from build123d import *

# Parameters (mm, degrees)
SKETCH1_R           = 3.175
BOSS_EXTRUDE1_DEPTH = 5.5499
FILLET1_START       = -5.5499
FILLET1_DEPTH       = 11.0998
SKETCH2_R           = 2.286
SKETCH2_R_2         = 1.89865
CUT_EXTRUDE1_DEPTH  = 5.08


with BuildPart() as part:
    # Sketch1 → Boss-Extrude1 (new, symmetric)
    with BuildSketch(Plane(origin=(0, 0, 0), x_dir=(1, 0, 0), z_dir=(0, 1, 0))):
        with BuildLine():
            Line((0, 6.35), (12.366459894, 6.35))
            Line((12.366459894, 6.35), (57.15, 6.35))
            Line((57.15, 6.35), (57.15, -3.81))
            Line((57.15, -3.81), (6.35, -3.81))
            Line((6.35, -3.81), (6.35, 0))
            ThreePointArc((6.35, 0), (-4.490128061, -4.490128061), (0, 6.35))
        make_face()
        with Locations(Location((0, 0, 0), (0, 0, 270))):
            Circle(SKETCH1_R, mode=Mode.SUBTRACT)
    extrude(amount=BOSS_EXTRUDE1_DEPTH, both=True)

    # Fillet1: read off the stored shape, not the designer's step
    # Fillet1 outline → Fillet1 (add)
    with BuildSketch(Plane(origin=(0, 0, 0), x_dir=(1, 0, 0), z_dir=(0, 1, 0)).offset(FILLET1_START)):
        with BuildLine():
            ThreePointArc((4.446322142, -4.533510716), (5.322474594, -3.972611562), (6.35, -3.81))
            Line((6.35, -3.81), (6.35, 0))
            ThreePointArc((6.35, 0), (5.854769236, -2.458490838), (4.446322142, -4.533510716))
        make_face()
    extrude(amount=FILLET1_DEPTH)

    # Sketch2 → Cut-Extrude1 (cut)
    with BuildSketch(Plane.XY.offset(3.81)):
        with Locations((13.97, 1.7399)):
            Circle(SKETCH2_R)
        with Locations((49.53, 1.7399)):
            Circle(SKETCH2_R)
        with Locations((13.97, 1.7399)):
            Circle(SKETCH2_R_2)
        with Locations((49.53, 1.7399)):
            Circle(SKETCH2_R_2)
    extrude(amount=-CUT_EXTRUDE1_DEPTH, mode=Mode.SUBTRACT)


solid = part.part
Can you work these out from the model? Positions are in its coordinate system, mm. A direction names the side the tool comes from. Give positions to 0.01 mm unless a question says otherwise; leave off trailing zeros. Order: outer loops, then holes, each group sorted by start corner. A loop starts at its lowest first (then second) coordinate and runs counter-clockwise, first axis right, second up. Notation, with made-up numbers: M -9.5,21 L 23.5,21 A23 ccw 23.5,40 Z; hole C 88,49 d11. An arc over 180 degrees is marked long. Use a Markdown table: item, result. Add a question column.
Item 1: We'd pull the mould along Z, two halves only. Please class faces 4 (the cylindrical face through (-5.81, 0.08, 2.56)), 5 (the flat face through (14, 2, -1.27)), 6 (the flat face through (25, -5.55, -2)), 7 (the cylindrical face through (-1.93, -0.08, -2.52)): +Z half, -Z half, draft (parallel to the pull), parting line (faces both ways), or undercut.
Item 2: Suppose I cut it at D-D (y = 1). List the corners of the cut face in (x, z) for me (3 decimals), then the cut area to 3 significant figures.
Item 3: If I drill on L1, parallel to Y at x = 13.97, z = 0.85; L2, parallel to X at y = 1, z = 0.75; L3, parallel to Z at x = 29, y = -4, over which ranges is the centre line in solid material (lowest first)? Write a range as [from, to].
Item 4: Suppose I cut it at B-B (z = 2.25). List the corners of the cut face in (x, y) for me, then the cut area to 3 significant figures.
Item 5: Suppose I cut it at A-A (y = 4.75). List the corners of the cut face in (x, z) for me (3 decimals), then the cut area to 3 significant figures.
Item 6: Suppose I cut it at C-C (x = 13.97). List the corners of the cut face in (y, z) for me.
Item 7: For faces 1 (the cylindrical face through (47.246, 1.84, 1.306)), 2 (the flat face through (25, 5.55, -2)), 3 (the flat face through (32, 0, 3.81)), which set-ups out of +Z, -Z, +X, -X, +Y, -Y let a thin tool reach every point of the face, with its end or its side?
Item 8: Will these pins go through, and if not, where does the flat tip stop? pin 1 (3 mm diameter, centred on y = -1, z = -2, fed in from -X); pin 2 (5 mm diameter, centred on x = 14, y = 2, fed in from +Z); pin 3 (5 mm diameter, centred on y = -2.5, z = -4.5, fed in from -X).
Answer sheet:
| question | item | result |
|---|---|---|
| 1 | face 4 | parting line |
| 1 | face 5 | +Z half |
| 1 | face 6 | draft |
| 1 | face 7 | undercut |
| 2 | outline | M 0,-6.35 L 57.15,-6.35 L 57.15,3.81 L 51.693,3.81 L 51.693,-1.27 L 47.367,-1.27 L 47.367,3.81 L 16.133,3.81 L 16.133,-1.27 L 11.807,-1.27 L 11.807,3.81 L 6.35,3.81 A2.54 cw 4.446,4.534 A6.35 ccw long Z; hole C 0,0 d6.35 |
| 2 | area | 578 mm² |
| 3 | L1 | y = [-5.55, -0.55], [4.03, 5.55] |
| 3 | L2 | x = [-6.31, -3.09], [3.09, 11.81], [16.13, 47.37], [51.69, 57.15] |
| 3 | L3 | z = [-6.35, 3.81] |
| 4 | outline | M -5.94,-5.55 L -2.24,-5.55 L -2.24,5.55 L -5.94,5.55 Z; M 2.24,-5.55 L 57.15,-5.55 L 57.15,5.55 L 2.24,5.55 Z; hole C 13.97,1.74 d4.57; hole C 49.53,1.74 d4.57 |
| 4 | area | 618 mm² |
| 5 | outline | M 0,-6.35 L 57.15,-6.35 L 57.15,3.81 L 6.35,3.81 A2.54 cw 4.446,4.534 A6.35 ccw long Z; hole C 0,0 d6.35 |
| 5 | area | 621 mm² |
| 6 | outline | M -5.55,-6.35 L 5.55,-6.35 L 5.55,3.81 L 4.03,3.81 L 4.03,-1.27 L -0.55,-1.27 L -0.55,3.81 L -5.55,3.81 Z |
| 7 | face 1 | +Z |
| 7 | face 2 | +Z, -Z, +X, -X, +Y |
| 7 | face 3 | +Z, +X, +Y, -Y |
| 8 | pin 1 | stops at x = -6.33 |
| 8 | pin 2 | stops at z = 3.81 |
| 8 | pin 3 | stops at x = -6.03 |
